Source: CAD feature listing. Evaluate the final solid. Frame: model axes, mm. Face numbers are marked on the shaded views. A direction names the side the tool comes from. Round coordinates to 2 decimals unless told otherwise and drop trailing zeros. Order: outer loops, then holes, each group sorted by start corner. A loop starts at its lowest first (then second) coordinate and runs counter-clockwise, first axis right, second up. Notation, with made-up numbers: (11, -40) -> (30, -40) arc R31 ccw to (30, -6) -> close; hole circle Ø3 at (26, -11). An arc over 180 degrees is marked (long way). One line per item, written item: value. Start each with the question number.
1) Reachability of the marked faces 5, 6 and 7 from +Z, -Z, +X, -X, +Y, -Y: full face, straight path, thin tool, end or side. Return the list, or none.
2) Section D-D (x = 36). Return the cut outline in (y, z).
3) Section A-A (x = 20). Return the cut outline in (y, z), and give its area (3 significant figures).
4) Ray query, L1, parallel to Y at x = 2, z = 6.5; L2, parallel to X at y = -15, z = 12; L3, parallel to Z at x = 18.5, y = -15. Return the intervals inside material, ascending.
5) Section B-B (y = -26). Return the cut outline in (x, z), and give its area (3 significant figures).
6) Mould query, pull axis Y, two halves, no side actions, for the marked faces 1, 2, 3 and 4. Classes: pulls with the +Y half, pulls with the -Y half, needs draft (parallel to the pull), parting line crosses it, or undercut.
7) Section C-C (z = 1.25). Return the cut outline in (x, y), and give its area (3 significant figures).
8) Pin query (flat end, axial travel): P1, Ø10, axis at x = 26, y = -6, coming from the -Z side; P2, Ø19, axis at x = 7.5, y = -15, coming from the -Z side; P3, Ø5, axis at x = 35, y = -27, coming from the -Z side. Return the tip coordinate at first contact, or that it passes through.
```python
from build123d import *

# Parameters (mm, degrees)
F0_R     = 2
F1_DEPTH = 4
F2_DEPTH = 34
F5_R     = 5


with BuildPart() as f1:
    # F0 (on Front) → F1 (new body)
    with BuildSketch(Plane.XZ):
        Polygon((0, 0), (0, 18), (40, 18), (40, 0), (40, -3), (43, -3), (43, 21), (-3, 21), (-3, -3), (0, -3), align=None)
        with BuildLine():
            Line((40, 18), (0, 18))
            Line((0, 18), (0, 0))
            Line((0, 0), (0, -3))
            Line((0, -3), (14.5, -3))
            ThreePointArc((14.5, -3), (20, -8.5), (25.5, -3))
            Line((25.5, -3), (40, -3))
            Line((40, -3), (40, 0))
            Line((40, 0), (40, 18))
        make_face()
        with Locations((20, -3)):
            Circle(F0_R, mode=Mode.SUBTRACT)
    extrude(amount=F1_DEPTH)

    # F0 (on Front) → F2 (join)
    with BuildSketch(Plane.XZ):
        Polygon((0, 0), (0, 18), (40, 18), (40, 0), (40, -3), (43, -3), (43, 21), (-3, 21), (-3, -3), (0, -3), align=None)
    extrude(amount=F2_DEPTH)

    # F4: F1 across plane


with BuildPart() as f1_1:
    add(f1.part)
    add(f1.part.mirror(Plane.XZ.offset(17)))

    # F5
    f5_edges = [f1_1.edges().sort_by_distance(p)[0] for p in [
        (20, 0, 21),
        (-3, -17, 21),
        (20, -34, 21),
        (43, -17, 21),
        (43, 0, 9),
        (-3, 0, 9),
        (-3, -34, 9),
        (43, -34, 9),
    ]]
    fillet(f5_edges, radius=F5_R)


solid = f1_1.part
```
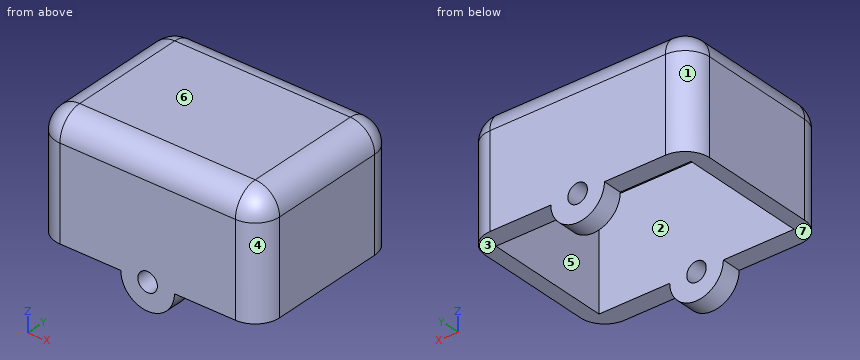
Findings:
1. face 5: -Z
1. face 6: +Z, +X, -X, +Y, -Y
1. face 7: -Z, -X, +Y, -Y
2. outline: (-34, -3) -> (-30, -3) -> (-30, 18) -> (-4, 18) -> (-4, -3) -> (0, -3) -> (0, 16) arc R5 ccw to (-5, 21) -> (-29, 21) arc R5 ccw to (-34, 16) -> close
3. outline: (-34, -8.5) -> (-30, -8.5) -> (-30, -5) -> (-34, -5) -> close; (-34, -1) -> (-30, -1) -> (-30, 18) -> (-4, 18) -> (-4, -1) -> (0, -1) -> (0, 16) arc R5 ccw to (-5, 21) -> (-29, 21) arc R5 ccw to (-34, 16) -> close; (-4, -8.5) -> (0, -8.5) -> (0, -5) -> (-4, -5) -> close
3. area: 271 mm2
4. L1: -34 to -30, -4 to 0
4. L2: -3 to 0, 40 to 43
4. L3: 18 to 21
5. outline: (-3, -3) -> (0, -3) -> (0, 18) -> (40, 18) -> (40, -3) -> (43, -3) -> (43, 16) arc R5 ccw to (38, 21) -> (2, 21) arc R5 ccw to (-3, 16) -> close
5. area: 253 mm2
6. face 1: pulls with the +Y half
6. face 2: undercut
6. face 3: needs draft
6. face 4: pulls with the -Y half
7. outline: (-3, -29) arc R5 ccw to (2, -34) -> (38, -34) arc R5 ccw to (43, -29) -> (43, -5) arc R5 ccw to (38, 0) -> (2, 0) arc R5 ccw to (-3, -5) -> close; hole (0, -30) -> (40, -30) -> (40, -4) -> (0, -4) -> close
7. area: 503 mm2
8. P1: z = -8.31
8. P2: z = -3
8. P3: z = 18
